from build123d import *

# Parameters (mm, degrees)
PCB_DEPTH       = 3
ESBO_O4_R       = 1.5
FUROS_PCB_DEPTH = 75.972458232


with BuildPart() as part:
    # Esboço3 → PCB (new body)
    with BuildSketch(Plane(origin=(0, 0, 0), x_dir=(0, 0, -1), z_dir=(1, 0, 0))):
        with BuildLine():
            Line((-1.863527408, 22.600091465), (38.136472592, 22.600091465))
            Line((38.136472592, 22.600091465), (38.136472592, 29.600091465))
            ThreePointArc((38.136472592, 29.600091465), (39.015152248, 31.721411809), (41.136472592, 32.600091465))
            Line((41.136472592, 32.600091465), (45.136472592, 32.600091465))
            ThreePointArc((45.136472592, 32.600091465), (47.257792935, 31.721411809), (48.136472592, 29.600091465))
            Line((48.136472592, 29.600091465), (48.136472592, 22.600091465))
            Line((48.136472592, 22.600091465), (48.136472592, -47.399908535))
            Line((48.136472592, -47.399908535), (48.136472592, -54.399908535))
            ThreePointArc((48.136472592, -54.399908535), (47.257792935, -56.521228878), (45.136472592, -57.399908535))
            Line((45.136472592, -57.399908535), (41.136472592, -57.399908535))
            ThreePointArc((41.136472592, -57.399908535), (39.015152248, -56.521228878), (38.136472592, -54.399908535))
            Line((38.136472592, -54.399908535), (38.136472592, -47.399908535))
            Line((38.136472592, -47.399908535), (-1.863527408, -47.399908535))
            Line((-1.863527408, -47.399908535), (-1.863527408, -54.399908535))
            ThreePointArc((-1.863527408, -54.399908535), (-2.742207065, -56.521228878), (-4.863527408, -57.399908535))
            Line((-4.863527408, -57.399908535), (-8.863527408, -57.399908535))
            ThreePointArc((-8.863527408, -57.399908535), (-10.984847752, -56.521228878), (-11.863527408, -54.399908535))
            Line((-11.863527408, -54.399908535), (-11.863527408, -47.399908535))
            Line((-11.863527408, -47.399908535), (-11.863527408, 22.600091465))
            Line((-11.863527408, 22.600091465), (-11.863527408, 29.600091465))
            ThreePointArc((-11.863527408, 29.600091465), (-10.984847752, 31.721411809), (-8.863527408, 32.600091465))
            Line((-8.863527408, 32.600091465), (-4.863527408, 32.600091465))
            ThreePointArc((-4.863527408, 32.600091465), (-2.742207065, 31.721411809), (-1.863527408, 29.600091465))
            Line((-1.863527408, 29.600091465), (-1.863527408, 22.600091465))
        make_face()
    extrude(amount=PCB_DEPTH)

    # Esboço4 → Furos PCB (cut, through all)
    with BuildSketch(Plane.ZY):
        with Locations((-43.136472592, 27.600091465)):
            Circle(ESBO_O4_R)
        with Locations((6.863527408, 27.600091465)):
            Circle(ESBO_O4_R)
        with Locations((6.863527408, -52.399908535)):
            Circle(ESBO_O4_R)
        with Locations((-43.136472592, -52.399908535)):
            Circle(ESBO_O4_R)
    extrude(amount=-FUROS_PCB_DEPTH, mode=Mode.SUBTRACT)


solid = part.part
CAD build for the part. Positions are in the model's coordinates, mm. A direction names the side the tool comes from. Give positions to 0.01 mm unless a question says otherwise; leave off trailing zeros. Order: outer loops, then holes, each group sorted by start corner. A loop starts at its lowest first (then second) coordinate and runs counter-clockwise, first axis right, second up. Notation, with made-up numbers: (46.25, 13) - (79.25, 13) arc R22 cw to (79.25, 21) - close; hole circle Ø7 at (14.25, -25). An arc over 180 degrees is marked (long way). Write each question's results on one line, items separated by ' | '.
1. Pin check, flat tips, straight feed: pin 1 (1.5 mm diameter, centred on x = 1, z = -25.5, fed in from +Y); pin 2 (0.9 mm diameter, centred on x = 1, z = -14, fed in from -Y). Stop position of each tip, or through.
Calculated:
pin 1: stops at y = 22.6 | pin 2: stops at y = -47.4
2. Probe L1, parallel to Z at x = 1.55, y = -49.5; L2, parallel to Y at x = 1.5, z = -42; L3, parallel to Y at x = 1.2, z = -44.5. List the from-to ranges inside material, lowest first. Write a range as from..to.
Calculated:
L1: z = -48.14..-38.14, 1.86..11.86 | L2: y = -57.4..-53.38, -51.42..26.62, 28.58..32.6 | L3: y = -57.4..-53.03, -51.77..26.97, 28.23..32.6
3. 3-axis set-ups, long thin cutter, end or side, ignore diameter. For faces 1 (the face through (1.479, 31.698, 11.008)), 2 (the face through (1, -51, 1.864)), 3 (the face through (1, 26, -38.136)): which of +Z, -Z, +X, -X, +Y, -Y reach the whole face in a straight line?
Calculated:
face 1: +Z, +X, -X, +Y | face 2: +X, -X, -Y | face 3: +X, -X, +Y
4. Saw through at B-B on x = 1.7. List the corners of the cut face in (y, z), and give its area (3 significant figures).
Calculated:
outline: (-57.4, -45.14) arc R3 ccw to (-54.4, -48.14) - (29.6, -48.14) arc R3 ccw to (32.6, -45.14) - (32.6, -41.14) arc R3 ccw to (29.6, -38.14) - (22.6, -38.14) - (22.6, 1.86) - (29.6, 1.86) arc R3 ccw to (32.6, 4.86) - (32.6, 8.86) arc R3 ccw to (29.6, 11.86) - (-54.4, 11.86) arc R3 ccw to (-57.4, 8.86) - (-57.4, 4.86) arc R3 ccw to (-54.4, 1.86) - (-47.4, 1.86) - (-47.4, -38.14) - (-54.4, -38.14) arc R3 ccw to (-57.4, -41.14) - close; hole circle Ø3 at (-52.4, -43.14); hole circle Ø3 at (-52.4, 6.86); hole circle Ø3 at (27.6, -43.14); hole circle Ø3 at (27.6, 6.86) | area: 4,560 mm2
5. Saw through at A-A on z = 7. List the corners of the cut face in (x, y), and give its area (3 significant figures).
Calculated:
outline: (0, -57.4) - (3, -57.4) - (3, -53.89) - (0, -53.89) - close; (0, -50.91) - (3, -50.91) - (3, 26.11) - (0, 26.11) - close; (0, 29.09) - (3, 29.09) - (3, 32.6) - (0, 32.6) - close | area: 252 mm2
6. Pull direction Z, two halves, no side cores. Call faces 4 (the face through (0, -12, -19)), 5 (the face through (1, -47.4, -18)), 6 (the face through (1, -13, 11.864)): released by +Z, released by -Z, zero draft, split by the parting line, or undercut.
Calculated:
face 4: zero draft | face 5: undercut | face 6: released by +Z
7. Saw through at C-C on z = -16. List the corners of the cut face in (x, y), and give its area (3 significant figures).
Calculated:
outline: (0, -47.4) - (3, -47.4) - (3, 22.6) - (0, 22.6) - close | area: 210 mm2
